Could you check a few things on this model? Use its own coordinates, in mm. A direction names the side the tool comes from. Give positions to 0.01 mm unless a question says otherwise; leave off trailing zeros. Write each loop counter-clockwise with the first axis right and the second up, starting at its lowest first coordinate (ties: lowest second). Pieces come first, ordered by that corner, then holes. Notation, with made-up numbers: (27, 20.25) - (47, 20.25) arc R13 ccw to (47, 38.25) - close; hole circle Ø1 at (66, -40). An arc over 180 degrees is marked (long way). Write item = value, one per line.
from build123d import *

# Parameters (mm, degrees)
SKETCH1_W               = 12.04
SKETCH1_H               = 7.58
SKETCH1_W_2             = 8.04
SKETCH1_H_2             = 3.58
BOSS_EXTRUDE1_DEPTH     = 8
SKETCH1_2_W             = 12.04
SKETCH1_2_H             = 7.58
SKETCH1_2_W_2           = 8.04
SKETCH1_2_H_2           = 3.58
BOSS_EXTRUDE2_DEPTH     = 2
EXTRUDE_THIN1_START     = -12.04
EXTRUDE_THIN1_DEPTH     = 12.04
SKETCH5_W               = 12.04
SKETCH5_H               = 7.58
SKETCH5_W_2             = 8.04
SKETCH5_H_2             = 3.58
BOSS_EXTRUDE4_DEPTH     = 10
SKETCH5_4_W             = 12.04
SKETCH5_4_H             = 7.58
BOSS_EXTRUDE5_DEPTH     = 2
CHAMFER1_SIZE           = 1.5
CUT_EXTRUDE1_DEPTH      = 29.028711337
CUT_EXTRUDE1_DEPTH_BACK = 29.028711337
CUT_EXTRUDE2_DEPTH      = 29.071269996
CUT_EXTRUDE2_DEPTH_BACK = 29.071269996
SKETCH8_W               = 4
SKETCH8_H               = 1.58
CUT_EXTRUDE3_DEPTH      = 6.5
SKETCH9_W               = 4
SKETCH9_H               = 1.58
CUT_EXTRUDE4_DEPTH      = 6.5
CHAMFER2_SIZE           = 0.5
BOSS_EXTRUDE8_DEPTH     = 0.3


with BuildPart() as part:
    # Sketch1 → Boss-Extrude1 (new body)
    with BuildSketch(Plane.XY):
        Rectangle(SKETCH1_W, SKETCH1_H)
        Rectangle(SKETCH1_W_2, SKETCH1_H_2, mode=Mode.SUBTRACT)
    extrude(amount=BOSS_EXTRUDE1_DEPTH)

    # Sketch1<2> → Boss-Extrude2 (add)
    # profile 1 of 2: a face of its own
    with BuildSketch(Plane.XY):
        Rectangle(SKETCH1_2_W, SKETCH1_2_H)
        Rectangle(SKETCH1_2_W_2, SKETCH1_2_H_2, mode=Mode.SUBTRACT)
    # profile 2 of 2: a face of its own
    with BuildSketch(Plane.XY):
        Rectangle(SKETCH1_2_W_2, SKETCH1_2_H_2)
    extrude(amount=-BOSS_EXTRUDE2_DEPTH)

    # Sketch3 → Extrude-Thin1 (add)
    with BuildSketch(Plane(origin=(6.02, 9.81, 0), x_dir=(0, -1, 0), z_dir=(1, 0, 0)).offset(EXTRUDE_THIN1_START)):
        with BuildLine():
            Line((13.6, 2), (9.52, 2))
            ThreePointArc((9.52, 2), (9.367259482, 9), (8.909328677, 15.986675107))
            Line((8.909328677, 15.986675107), (12.973803045, 16.342270537))
            Line((12.973803045, 16.342270537), (12.799491559, 18.334659933))
            Line((12.799491559, 18.334659933), (6.730055387, 17.803653074))
            ThreePointArc((6.730055387, 17.803653074), (7.369163038, 8.912761225), (7.507379539, 0))
            Line((7.507379539, 0), (13.6, 0))
            Line((13.6, 0), (13.6, 2))
        make_face()
    extrude(amount=EXTRUDE_THIN1_DEPTH)

    # Sketch5 → Boss-Extrude4 (add)
    with BuildSketch(Plane(origin=(0, -2.356055999, -16.271601827), x_dir=(-1, 0, 0), z_dir=(0, 0.08715574274765182, -0.9961946980917462))):
        with Locations((0, 2.979167492)):
            Rectangle(SKETCH5_W, SKETCH5_H)
        with Locations((0, 2.979167492)):
            Rectangle(SKETCH5_W_2, SKETCH5_H_2, mode=Mode.SUBTRACT)
    extrude(amount=BOSS_EXTRUDE4_DEPTH)

    # Sketch5<4> → Boss-Extrude5 (add)
    with BuildSketch(Plane(origin=(0, -2.356055999, -16.271601827), x_dir=(-1, 0, 0), z_dir=(0, 0.08715574274765182, -0.9961946980917462))):
        with Locations((0, 2.979167492)):
            Rectangle(SKETCH5_4_W, SKETCH5_4_H)
    extrude(amount=BOSS_EXTRUDE5_DEPTH)

    # Chamfer1
    chamfer1_edges = [part.edges().sort_by_distance(p)[0] for p in [
        (0, -3.79, -2),
        (0, 3.79, -2),
        (-6.02, -2.728024331, -21.323244027),
        (6.02, -2.728024331, -21.323244027),
        (0, -3.163803045, -16.342270537),
        (6.02, -3.79, 3),
        (-6.02, -3.79, 3),
        (-6.02, 3.79, 3),
        (6.02, 3.79, 3),
        (0, 4.387352767, -15.681630007),
        (6.02, 4.82313148, -20.662603497),
        (-6.02, 4.82313148, -20.662603497),
    ]]
    chamfer(chamfer1_edges, length=CHAMFER1_SIZE - 0.0001)  # a hair under: the kernel refuses the full size

    # Sketch6 → Cut-Extrude1 (cut, two sides: drawn at the far end of the back side and taken through both)
    with BuildSketch(Plane(origin=(0, 3.79, 0), x_dir=(1, 0, 0), z_dir=(0, 1, 0)).offset(-CUT_EXTRUDE1_DEPTH_BACK)):
        with BuildLine():
            Line((1.05, -3.393782217), (0, -2.787564435))
            ThreePointArc((0, -2.787564435), (-0.7, -2.787564435), (-1.05, -3.393782217))
            Line((-1.05, -3.393782217), (-1.05, -4.606217783))
            ThreePointArc((-1.05, -4.606217783), (-0.7, -5.212435565), (0, -5.212435565))
            Line((0, -5.212435565), (1.05, -4.606217783))
            ThreePointArc((1.05, -4.606217783), (1.4, -4), (1.05, -3.393782217))
        make_face()
    extrude(amount=CUT_EXTRUDE1_DEPTH + CUT_EXTRUDE1_DEPTH_BACK, mode=Mode.SUBTRACT)

    # Sketch7 → Cut-Extrude2 (cut, two sides: drawn at the far end of the back side and taken through both)
    with BuildSketch(Plane(origin=(0, 2.992482656, 0.261808308), x_dir=(1, 0, 0), z_dir=(0, 0.9961946980917462, 0.08715574274765181)).offset(-CUT_EXTRUDE2_DEPTH_BACK)):
        with BuildLine():
            Line((1.05, 22.610557442), (0, 23.216775225))
            ThreePointArc((0, 23.216775225), (-0.7, 23.216775225), (-1.05, 22.610557442))
            Line((-1.05, 22.610557442), (-1.05, 21.398121877))
            ThreePointArc((-1.05, 21.398121877), (-0.7, 20.791904094), (0, 20.791904094))
            Line((0, 20.791904094), (1.05, 21.398121877))
            ThreePointArc((1.05, 21.398121877), (1.4, 22.004339659), (1.05, 22.610557442))
        make_face()
    extrude(amount=CUT_EXTRUDE2_DEPTH + CUT_EXTRUDE2_DEPTH_BACK, mode=Mode.SUBTRACT)

    # Sketch8 → Cut-Extrude3 (cut)
    with BuildSketch(Plane(origin=(0, 2.266427538, -25.905385296), x_dir=(-1, 0, 0), z_dir=(0, 0.08715574274765193, -0.9961946980917461))):
        with Locations((-6.02, -0.786086546)):
            Rectangle(SKETCH8_W, SKETCH8_H)
    extrude(amount=-CUT_EXTRUDE3_DEPTH, mode=Mode.SUBTRACT)

    # Sketch9 → Cut-Extrude4 (cut)
    with BuildSketch(Plane.XY.offset(8)):
        with Locations((6.02, 0)):
            Rectangle(SKETCH9_W, SKETCH9_H)
    extrude(amount=-CUT_EXTRUDE4_DEPTH, mode=Mode.SUBTRACT)

    # Chamfer2
    chamfer2_edges = [part.edges().sort_by_distance(p)[0] for p in [
        (4.02, 0.413082313, -22.805117521),
        (4.02, 0.91681996, -19.498631715),
        (4.02, 1.987069936, -22.667411447),
        (4.02, 0.79, 4.75),
        (4.02, 0, 1.5),
        (4.02, -0.79, 4.75),
    ]]
    chamfer(chamfer2_edges, length=CHAMFER2_SIZE)

    # Sketch12 → Boss-Extrude8 (add)
    with BuildSketch(Plane(origin=(6.02, 0, 0), x_dir=(0, 0, -1), z_dir=(1, 0, 0))):
        Polygon((17.914805855, 1.992834285), (18.088967441, 0.000456236), (17.664424758, -0.036510227), (17.490263173, 1.955867821), align=None)
    extrude(amount=BOSS_EXTRUDE8_DEPTH)


solid = part.part
1. If we section it at D-D, the plane z = -10: Please give me the cut outline in (x, y).
Filled sheet:
outline = (-6.02, 0.49) - (6.02, 0.49) - (6.02, 2.49) - (-6.02, 2.49) - close
2. If we section it at C-C, the plane z = -20: Please give me the cut outline in (x, y), and give its area (3 significant figures).
Filled sheet:
outline = (-6.02, -1.34) - (-4.52, -2.84) - (4.52, -2.84) - (6.02, -1.34) - (6.02, 0.17) - (4.52, 0.17) - (4.02, -0.33) - (4.02, -0.84) - (-4.02, -0.84) - (-4.02, 2.76) - (4.02, 2.76) - (4.02, 2.26) - (4.52, 1.75) - (6.02, 1.75) - (6.02, 3.26) - (4.52, 4.77) - (-4.52, 4.77) - (-6.02, 3.26) - close
area = 54.8 mm2
3. If we section it at A-A, the plane z = 4: Please give me the cut outline in (x, y).
Filled sheet:
outline = (-6.02, -2.29) - (-4.52, -3.79) - (-1.05, -3.79) - (-1.05, -1.79) - (-4.02, -1.79) - (-4.02, 1.79) - (-1.05, 1.79) - (-1.05, 3.79) - (-4.52, 3.79) - (-6.02, 2.29) - close; (1.4, -3.79) - (4.52, -3.79) - (6.02, -2.29) - (6.02, -0.79) - (4.52, -0.79) - (4.02, -1.29) - (4.02, -1.79) - (1.4, -1.79) - close; (1.4, 1.79) - (4.02, 1.79) - (4.02, 1.29) - (4.52, 0.79) - (6.02, 0.79) - (6.02, 2.29) - (4.52, 3.79) - (1.4, 3.79) - close
4. For pin 1 (1 mm diameter, centred on x = -0.5, z = -20, fed in from +Y) (3 decimals); pin 2 (0.8 mm diameter, centred on x = 5.5, z = 5.5, fed in from -Y); pin 3 (4 mm diameter, centred on y = 1, z = -12.5, fed in from +X), each with a flat end and sliding along its axis, tell me the tip position at first contact or that it passes through.
Filled sheet:
pin_1 = 4.805
pin_2 = -3.21
pin_3 = 6.02
5. Which directions (+Z, -Z, +X, -X, +Y, -Y) give clear straight access to the entire face, cutting with the end or side of a thin tool? Please do faces 4 (the face through (5, -0.79, 5)), 5 (the face through (-0.084, 2.445, -9.009)), 6 (the face through (1, 1.79, 5)), 7 (the face through (-0.709, -2.804, 5.207)), 8 (the face through (0.95, 2.836, -20.892)).
Filled sheet:
face_4 = +Z, +X
face_5 = +X, -X, +Y
face_6 = +Z
face_7 = +Y, -Y
face_8 = -Z
6. Thinking about a two-plate mould opening in X: for faces 1 (the face through (-5.26, 4.09, -20.8)), 2 (the face through (0, 0, 0)), 3 (the face through (-0.08, -2.34, -17.01)), which applies, pulls with the +X half, pulls with the -X half, needs draft (parallel to the pull), parting line crosses it, or undercut?
Filled sheet:
face_1 = pulls with the -X half
face_2 = undercut
face_3 = needs draft
7. I need wall thicknesses on line 1 (Y direction, x = -1.25, z = 4.5); line 2 (Z direction, x = -0.5, y = -1.25); line 3 (X direction, y = -1.25, z = 0.5). Which ranges of each line are inside material? Lowest first, please.
Filled sheet:
line_1 = -3.79 to -1.79, 1.79 to 3.79
line_2 = -26.21 to -23.49, -20.9 to -16.17, -2 to 0
line_3 = -6.02 to -4.02, 4.02 to 6.02
